Input: part model. Units: mm. Frame: model coordinates. Coordinates: 2 decimals unless noted, no trailing zeros. Order: outer loops, then holes, each group sorted by start corner. A loop starts at its lowest first (then second) coordinate and runs counter-clockwise, first axis right, second up.
from build123d import *

# Parameters (mm, degrees)
SKETCH2_W           = 177.8
SKETCH2_H           = 177.8
BOSS_EXTRUDE1_DEPTH = 6.35
SKETCH3_R           = 2.5
CUT_EXTRUDE1_DEPTH  = 12.7
CUT_EXTRUDE2_REACH  = 128.363
SKETCH5_R           = 3.175


with BuildPart() as part:
    # Sketch2 → Boss-Extrude1 (new, symmetric)
    with BuildSketch(Plane(origin=(0, 0, 0), x_dir=(1, 0, 0), z_dir=(0, 1, 0))):
        Rectangle(SKETCH2_W, SKETCH2_H)
        with BuildLine():
            Line((-1.8, 2.4), (1.8, 2.4))
            ThreePointArc((1.8, 2.4), (0, -3), (-1.8, 2.4))
        make_face(mode=Mode.SUBTRACT)
    extrude(amount=BOSS_EXTRUDE1_DEPTH, both=True)

    # Sketch3 → Cut-Extrude1 (cut)
    with BuildSketch(Plane.XZ.offset(6.35)):
        with Locations(Location((-59.856589027, -59.856589027, 0), (0, 0, 270))):
            Circle(SKETCH3_R)
        with Locations(Location((59.856589027, -59.856589027, 0), (0, 0, 270))):
            Circle(SKETCH3_R)
        with Locations(Location((59.856589027, 59.856589027, 0), (0, 0, 270))):
            Circle(SKETCH3_R)
        with Locations(Location((-59.856589027, 59.856589027, 0), (0, 0, 270))):
            Circle(SKETCH3_R)
    extrude(amount=-CUT_EXTRUDE1_DEPTH, mode=Mode.SUBTRACT)

    # Sketch5 → Cut-Extrude2 (cut, up to next)
    with BuildSketch(Plane(origin=(0, 6.35, 0), x_dir=(1, 0, 0), z_dir=(0, 1, 0)), mode=Mode.PRIVATE) as cut_extrude2_sk1:
        with Locations(Location((20.113342208, -6.35, 0), (0, 0, 270))):
            Circle(SKETCH5_R)
    cut_extrude2_tool1 = extrude(cut_extrude2_sk1.sketch, amount=-CUT_EXTRUDE2_REACH, mode=Mode.PRIVATE) & part.part
    # Sketch5 → Cut-Extrude2 (cut, up to next)
    with BuildSketch(Plane(origin=(0, 6.35, 0), x_dir=(1, 0, 0), z_dir=(0, 1, 0)), mode=Mode.PRIVATE) as cut_extrude2_sk2:
        with Locations(Location((-29.035657792, -21.552614691, 0), (0, 0, 270))):
            Circle(SKETCH5_R)
    cut_extrude2_tool2 = extrude(cut_extrude2_sk2.sketch, amount=-CUT_EXTRUDE2_REACH, mode=Mode.PRIVATE) & part.part
    add(cut_extrude2_tool1.solids().sort_by_distance((20.113342, 6.35, 6.35))[0], mode=Mode.SUBTRACT)
    add(cut_extrude2_tool2.solids().sort_by_distance((-29.035658, 6.35, 21.552615))[0], mode=Mode.SUBTRACT)


solid = part.part
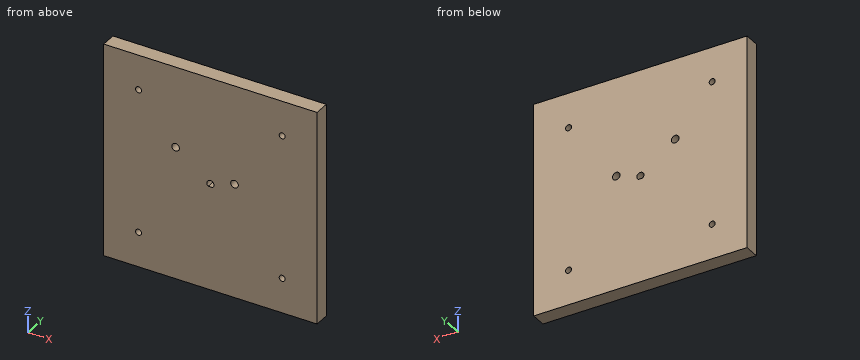
Item 1: Pin query (flat end, axial travel): pin 1 Ø4.5 at (x, z) = (59.86, -59.86) entering from +Y. Return the tip coordinate at first contact, or that it passes through.
Response values:
pin 1: passes through
Item 2: Ray query, probe 1 along X at (y, z) = (-5.5, -60); probe 2 along Z at (x, y) = (0, -3.5); probe 3 along X at (y, z) = (-0.75, -58.5). Return the intervals inside material, ascending.
Response values:
probe 1: x = -88.9 to -62.35, -57.36 to 57.36, 62.35 to 88.9
probe 2: z = -88.9 to -2.4, 3 to 88.9
probe 3: x = -88.9 to -61.96, -57.76 to 57.76, 61.96 to 88.9
Item 3: Cut plane A-A on z = 0. Return loops of the section in (x, y), then the cut area to 3 significant figures.
Response values:
outline: (-88.9, -6.35) - (-3, -6.35) - (-3, 6.35) - (-88.9, 6.35) - close; (3, -6.35) - (88.9, -6.35) - (88.9, 6.35) - (3, 6.35) - close
area: 2,180 mm2
